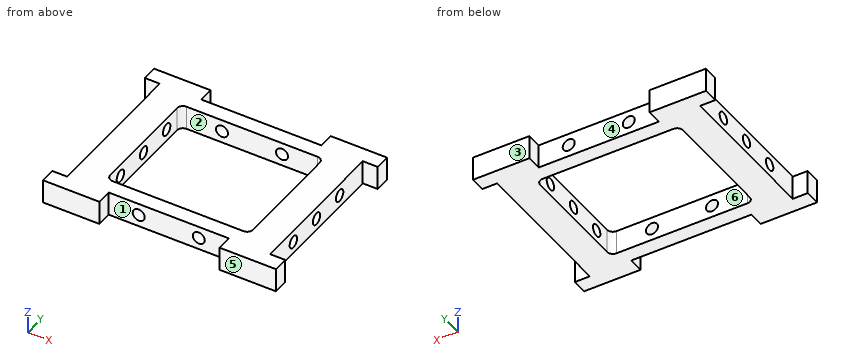
from build123d import *

# Parameters (mm, degrees)
SKETCH_1_W          = 67.6
SKETCH_1_H          = 50
EXTRUDE_1_DEPTH     = 8
SKETCH_2_R          = 2
CUT_EXTRUDE_1_DEPTH = 10
SKETCH_3_R          = 2
CUT_EXTRUDE_2_DEPTH = 10
SKETCH_4_W          = 18.8
SKETCH_4_H          = 5
EXTRUDE_2_DEPTH     = 8
SKETCH_5_W          = 47.6
SKETCH_5_H          = 40
CUT_EXTRUDE_3_DEPTH = 8
FILLET_1_R          = 2


with BuildPart() as part:
    # 草图1 → 凸台-拉伸1 (new body)
    with BuildSketch(Plane.XY):
        with Locations((33.8, 25)):
            Rectangle(SKETCH_1_W, SKETCH_1_H)
    extrude(amount=EXTRUDE_1_DEPTH)

    # 草图2 → 切除-拉伸1 (cut)
    with BuildSketch(Plane.ZY):
        with Locations((4, 37.5)):
            Circle(SKETCH_2_R)
        with Locations((4, 25)):
            Circle(SKETCH_2_R)
        with Locations((4, 12.5)):
            Circle(SKETCH_2_R)
    cut_extrude_1 = extrude(amount=-CUT_EXTRUDE_1_DEPTH, mode=Mode.SUBTRACT)

    # 镜向1: 切除-拉伸1 across plane
    add(cut_extrude_1.mirror(Plane(origin=(33.8, 0, 0), x_dir=(0, 0, 1), z_dir=(1, 0, 0))), mode=Mode.SUBTRACT)

    # 草图3 → 切除-拉伸2 (cut)
    with BuildSketch(Plane(origin=(0, 50, 0), x_dir=(1, 0, 0), z_dir=(0, 1, 0))):
        with Locations(Location((23.8, -4, 0), (0, 0, 270))):
            Circle(SKETCH_3_R)
        with Locations(Location((43.8, -4, 0), (0, 0, 270))):
            Circle(SKETCH_3_R)
    cut_extrude_2 = extrude(amount=-CUT_EXTRUDE_2_DEPTH, mode=Mode.SUBTRACT)

    # 镜向2: 切除-拉伸2 across plane
    add(cut_extrude_2.mirror(Plane.ZX.offset(25)), mode=Mode.SUBTRACT)

    # 草图4 → 凸台-拉伸2 (add)
    with BuildSketch(Plane(origin=(0, 0, 0), x_dir=(-1, 0, 0), z_dir=(0, 0, -1))):
        with Locations((-63.2, 52.5)):
            Rectangle(SKETCH_4_W, SKETCH_4_H)
        with Locations((-63.2, -2.5)):
            Rectangle(SKETCH_4_W, SKETCH_4_H)
        with Locations((-4.4, -2.5)):
            Rectangle(SKETCH_4_W, SKETCH_4_H)
        with Locations((-4.4, 52.5)):
            Rectangle(SKETCH_4_W, SKETCH_4_H)
    extrude(amount=-EXTRUDE_2_DEPTH)

    # 草图5 → 切除-拉伸3 (cut)
    with BuildSketch(Plane(origin=(0, 0, 0), x_dir=(-1, 0, 0), z_dir=(0, 0, -1))):
        with Locations((-33.8, 25)):
            Rectangle(SKETCH_5_W, SKETCH_5_H)
    extrude(amount=-CUT_EXTRUDE_3_DEPTH, mode=Mode.SUBTRACT)

    # 圆角1
    fillet_1_edges = [part.edges().sort_by_distance(p)[0] for p in [
        (10, 45, 4),
        (57.6, 45, 4),
        (57.6, 5, 4),
        (10, 5, 4),
    ]]
    fillet(fillet_1_edges, radius=FILLET_1_R)


solid = part.part
Source: CAD feature listing. Evaluate the final solid. Frame: model axes, mm. Face numbers are marked on the shaded views. A direction names the side the tool comes from. Give positions to 0.01 mm unless a question says otherwise; leave off trailing zeros. Write each loop counter-clockwise with the first axis right and the second up, starting at its lowest first coordinate (ties: lowest second). Pieces come first, ordered by that corner, then holes. Notation, with made-up numbers: (80.25, -25.5) -> (117.25, -25.5) arc R13 ccw to (117.25, -1.5) -> close; hole circle Ø2 at (-0.5, -0.5). An arc over 180 degrees is marked (long way). Return JSON: item names as keys, results as strings. Group by question number.
1. Section B-B, the plane z = 7. Output: boundary loops of the cut face in (x, y).
2. Section C-C, the plane y = 37.5. Output: boundary loops of the cut face in (x, z), then the cut area to 3 significant figures.
3. Material intervals for line 1 (X direction, y = 3.9, z = 4); line 2 (Y direction, x = 60.75, z = 4); line 3 (Z direction, x = 43.8, y = 2.2), sorted ascending. Write a range as from..to.
4. Mould query, pull axis Y, two halves, no side actions, for the marked faces 4, 5 and 6. Classes: +Y half, -Y half, draft (parallel to the pull), parting line (faces both ways), or undercut.
5. Access query for the marked faces 1, 2 and 3. Directions: +Z, -Z, +X, -X, +Y, -Y. A direction counts if a zero-diameter tool reaches every point of the face in a straight line with its end or side. Return the directions, or none.
6. Section D-D, the plane x = 23.8. Output: boundary loops of the cut face in (y, z).
7. Section A-A, the plane x = 15. Output: boundary loops of the cut face in (y, z).
8. Pin query (flat end, axial travel): pin 1 Ø4 at (x, z) = (26.5, 3) entering from -Y; pin 2 Ø4 at (y, z) = (28, 2.5) entering from +X; pin 3 Ø3 at (y, z) = (42, 5) entering from -X. Return the tip coordinate at first contact, or that it passes through.
Determined:
{
 "1": {"outline": "(-5, -5) -> (13.8, -5) -> (13.8, 0) -> (53.8, 0) -> (53.8, -5) -> (72.6, -5) -> (72.6, 0) -> (67.6, 0) -> (67.6, 50) -> (72.6, 50) -> (72.6, 55) -> (53.8, 55) -> (53.8, 50) -> (13.8, 50) -> (13.8, 55) -> (-5, 55) -> (-5, 50) -> (0, 50) -> (0, 0) -> (-5, 0) -> close; hole (10, 7) arc R2 ccw to (12, 5) -> (55.6, 5) arc R2 ccw to (57.6, 7) -> (57.6, 43) arc R2 ccw to (55.6, 45) -> (12, 45) arc R2 ccw to (10, 43) -> close"},
 "2": {"outline": "(0, 0) -> (10, 0) -> (10, 2) -> (0, 2) -> close; (0, 6) -> (10, 6) -> (10, 8) -> (0, 8) -> close; (57.6, 0) -> (67.6, 0) -> (67.6, 2) -> (57.6, 2) -> close; (57.6, 6) -> (67.6, 6) -> (67.6, 8) -> (57.6, 8) -> close", "area": "80.0 mm2"},
 "3": {"line 1": "x = 0..21.8, 25.8..41.8, 45.8..67.6", "line 2": "y = -5..10.5, 14.5..23, 27..35.5, 39.5..55", "line 3": "z = 0..2, 6..8"},
 "4": {"face 4": "+Y half", "face 5": "-Y half", "face 6": "undercut"},
 "5": {"face 1": "+Z, -Z, -Y", "face 2": "+Z, -Z", "face 3": "+Z, -Z, +X, -X, +Y"},
 "6": {"outline": "(0, 0) -> (5, 0) -> (5, 2) -> (0, 2) -> close; (0, 6) -> (5, 6) -> (5, 8) -> (0, 8) -> close; (45, 0) -> (50, 0) -> (50, 2) -> (45, 2) -> close; (45, 6) -> (50, 6) -> (50, 8) -> (45, 8) -> close"},
 "7": {"outline": "(0, 0) -> (5, 0) -> (5, 8) -> (0, 8) -> close; (45, 0) -> (50, 0) -> (50, 8) -> (45, 8) -> close"},
 "8": {"pin 1": "stops at y = 0", "pin 2": "stops at x = 67.6", "pin 3": "stops at x = 0"}
}
